Check sheet for the modelled part. Datum: model origin and axes. Units: mm. Round coordinates to 2 decimals unless told otherwise and drop trailing zeros. Loops run counter-clockwise (first coordinate to the right, second up) from the corner with the lowest first, then second, coordinate; pieces in that order, holes last. Notation, with made-up numbers: (57.25, 40.5) - (71.25, 40.5) arc R10 cw to (71.25, 49.5) - close; hole circle Ø7 at (63.5, 69.5). An arc over 180 degrees is marked (long way). Return JSON: item names as keys, results as strings.
from build123d import *

# Parameters (mm, degrees)
F0_W     = 596.9
F0_H     = 587.3496
F0_R     = 25.4
F1_DEPTH = 4.7752
F2_R     = 38.1
F3_W     = 146.05
F3_H     = 6.35
F4_DEPTH = 25.4


with BuildPart() as f1:
    # F0 (on Top) → F1 (new body)
    with BuildSketch(Plane.XY):
        with Locations((298.45, 293.6748)):
            Rectangle(F0_W, F0_H)
        with Locations((63.5, 63.5)):
            Circle(F0_R, mode=Mode.SUBTRACT)
        with Locations((157.48, 63.5)):
            Circle(F0_R, mode=Mode.SUBTRACT)
        with Locations((251.46, 63.5)):
            Circle(F0_R, mode=Mode.SUBTRACT)
        with Locations((63.5, 152.4)):
            Circle(F0_R, mode=Mode.SUBTRACT)
        with Locations((63.5, 241.3)):
            Circle(F0_R, mode=Mode.SUBTRACT)
        with Locations((157.48, 152.4)):
            Circle(F0_R, mode=Mode.SUBTRACT)
        with Locations((251.46, 152.4)):
            Circle(F0_R, mode=Mode.SUBTRACT)
        with Locations((157.48, 241.3)):
            Circle(F0_R, mode=Mode.SUBTRACT)
        with Locations((251.46, 241.3)):
            Circle(F0_R, mode=Mode.SUBTRACT)
        with Locations((345.44, 63.5)):
            Circle(F0_R, mode=Mode.SUBTRACT)
        with Locations((439.42, 63.5)):
            Circle(F0_R, mode=Mode.SUBTRACT)
        with Locations((533.4, 63.5)):
            Circle(F0_R, mode=Mode.SUBTRACT)
        with Locations((345.44, 152.4)):
            Circle(F0_R, mode=Mode.SUBTRACT)
        with Locations((439.42, 152.4)):
            Circle(F0_R, mode=Mode.SUBTRACT)
        with Locations((345.44, 241.3)):
            Circle(F0_R, mode=Mode.SUBTRACT)
        with Locations((439.42, 241.3)):
            Circle(F0_R, mode=Mode.SUBTRACT)
        with Locations((533.4, 152.4)):
            Circle(F0_R, mode=Mode.SUBTRACT)
        with Locations((533.4, 241.3)):
            Circle(F0_R, mode=Mode.SUBTRACT)
        with Locations((63.5, 346.0496)):
            Circle(F0_R, mode=Mode.SUBTRACT)
        with Locations((63.5, 434.9496)):
            Circle(F0_R, mode=Mode.SUBTRACT)
        with Locations((157.48, 346.0496)):
            Circle(F0_R, mode=Mode.SUBTRACT)
        with Locations((251.46, 346.0496)):
            Circle(F0_R, mode=Mode.SUBTRACT)
        with Locations((157.48, 434.9496)):
            Circle(F0_R, mode=Mode.SUBTRACT)
        with Locations((251.46, 434.9496)):
            Circle(F0_R, mode=Mode.SUBTRACT)
        with Locations((63.5, 523.8496)):
            Circle(F0_R, mode=Mode.SUBTRACT)
        with Locations((157.48, 523.8496)):
            Circle(F0_R, mode=Mode.SUBTRACT)
        with Locations((251.46, 523.8496)):
            Circle(F0_R, mode=Mode.SUBTRACT)
        with Locations((345.44, 346.0496)):
            Circle(F0_R, mode=Mode.SUBTRACT)
        with Locations((439.42, 346.0496)):
            Circle(F0_R, mode=Mode.SUBTRACT)
        with Locations((345.44, 434.9496)):
            Circle(F0_R, mode=Mode.SUBTRACT)
        with Locations((439.42, 434.9496)):
            Circle(F0_R, mode=Mode.SUBTRACT)
        with Locations((533.4, 346.0496)):
            Circle(F0_R, mode=Mode.SUBTRACT)
        with Locations((533.4, 434.9496)):
            Circle(F0_R, mode=Mode.SUBTRACT)
        with Locations((345.44, 523.8496)):
            Circle(F0_R, mode=Mode.SUBTRACT)
        with Locations((439.42, 523.8496)):
            Circle(F0_R, mode=Mode.SUBTRACT)
        with Locations((533.4, 523.8496)):
            Circle(F0_R, mode=Mode.SUBTRACT)
    extrude(amount=F1_DEPTH)

    # F2
    f2_edges = [f1.edges().sort_by_distance(p)[0] for p in [
        (0, 0, 2.3876),
        (596.9, 0, 2.3876),
        (596.9, 587.3496, 2.3876),
        (0, 587.3496, 2.3876),
    ]]
    fillet(f2_edges, radius=F2_R)

    # F3 (on face) → F4 (cut)
    with BuildSketch(Plane.XY.offset(4.7752)):
        with Locations((152.4, 293.6748)):
            Rectangle(F3_W, F3_H)
        with Locations((444.5, 293.6748)):
            Rectangle(F3_W, F3_H)
    extrude(amount=-F4_DEPTH, mode=Mode.SUBTRACT)


solid = f1.part
Q1. Sectioned sample at C-C (x = 332.5). Enter the section's corners in (y, z).
Answer key:
{"outline": "(0, 0) - (41.64, 0) - (41.64, 4.78) - (0, 4.78) - close; (85.36, 0) - (130.54, 0) - (130.54, 4.78) - (85.36, 4.78) - close; (174.26, 0) - (219.44, 0) - (219.44, 4.78) - (174.26, 4.78) - close; (263.16, 0) - (324.19, 0) - (324.19, 4.78) - (263.16, 4.78) - close; (367.91, 0) - (413.09, 0) - (413.09, 4.78) - (367.91, 4.78) - close; (456.81, 0) - (501.99, 0) - (501.99, 4.78) - (456.81, 4.78) - close; (545.71, 0) - (587.35, 0) - (587.35, 4.78) - (545.71, 4.78) - close"}
Q2. Sectioned sample at B-B (y = 63.5). Enter the section's corners in (x, z), plus the area to 3 significant figures.
Answer key:
{"outline": "(0, 0) - (38.1, 0) - (38.1, 4.78) - (0, 4.78) - close; (88.9, 0) - (132.08, 0) - (132.08, 4.78) - (88.9, 4.78) - close; (182.88, 0) - (226.06, 0) - (226.06, 4.78) - (182.88, 4.78) - close; (276.86, 0) - (320.04, 0) - (320.04, 4.78) - (276.86, 4.78) - close; (370.84, 0) - (414.02, 0) - (414.02, 4.78) - (370.84, 4.78) - close; (464.82, 0) - (508, 0) - (508, 4.78) - (464.82, 4.78) - close; (558.8, 0) - (596.9, 0) - (596.9, 4.78) - (558.8, 4.78) - close", "area": "1,390 mm²"}
Q3. Depth check by flat-ended pin: P1, Ø3, axis at x = 284, y = 129.5, coming from the -Z side. Enter the tip coordinate at first touch or a pass-through.
Answer key:
{"P1": "stops at z = 0"}
Q4. Draft check along Y on faces 1 (the face through (294, 298, 4.775)), 2 (the face through (245.954, 410.154, 2.354)), 3 (the face through (10.86, 11.46, 2.42)), 4 (the face through (180.943, 231.572, 2.354)). Enter one of: released by +Y, released by -Y, zero draft, split by the parting line, or undercut.
Answer key:
{"face 1": "zero draft", "face 2": "undercut", "face 3": "released by -Y", "face 4": "undercut"}
Q5. Sectioned sample at A-A (x = 157.48). State how many separate pieces and enclosed holes the cut face has, plus the area to 3 significant figures.
Answer key:
{"separate pieces": "8", "enclosed holes": "0", "area": "1,320 mm²"}
Q6. Scan lines: probe 1 along Y at (x, z) = (378, 1.05); probe 2 along Y at (x, z) = (27, 2.6). Record each from-to range of solid material in increasing order. Write a range as [from, to].
Answer key:
{"probe 1": "y = [0, 290.5], [296.85, 587.35]", "probe 2": "y = [1.65, 585.7]"}
